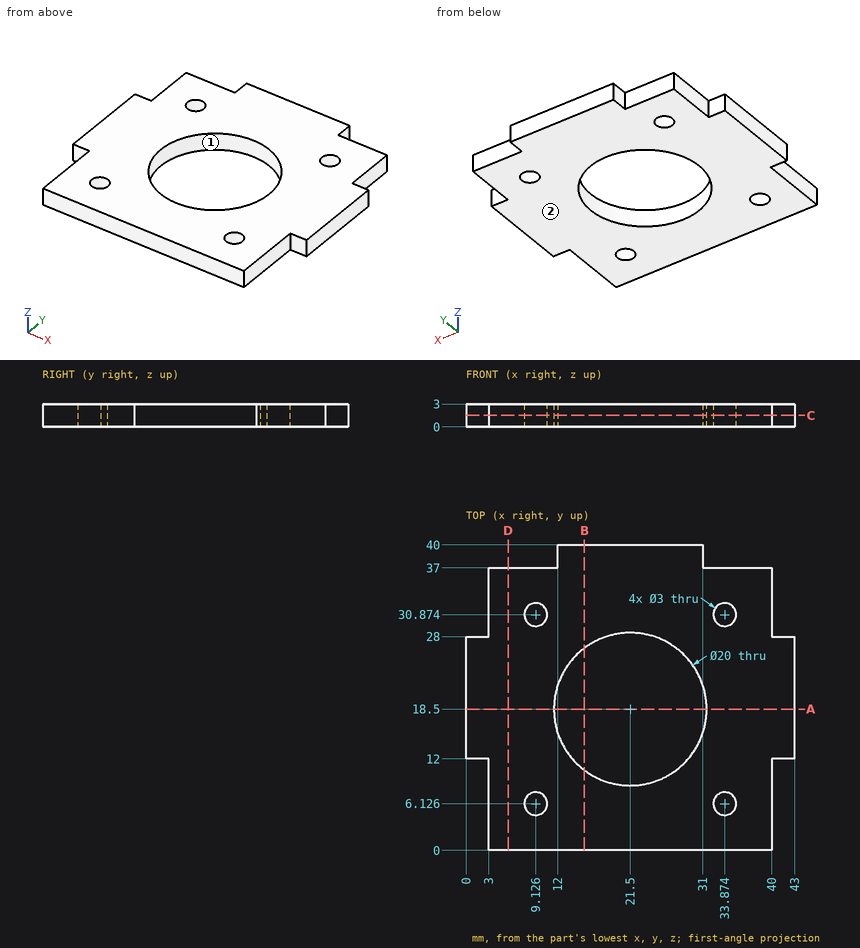
Input: dimensioned drawing with shaded views. Units: mm. Origin: part minimum x, y, z. Round coordinates to 2 decimals unless told otherwise and drop trailing zeros. Loops run counter-clockwise (first coordinate to the right, second up) from the corner with the lowest first, then second, coordinate; pieces in that order, holes last.
1) Pull-direction query (X, two-part tool) for the marked faces 1 and 2; classes: released by +X, released by -X, zero draft, split by the parting line, or undercut.
Ans:
face 1: undercut
face 2: zero draft
2) Pin query (flat end, axial travel): pin 1 (1.5 mm diameter, centred on x = 1.5, z = 1.5, fed in from -Y); pin 2 (1.5 mm diameter, centred on y = 38, z = 1.5, fed in from +X); pin 3 (0.9 mm diameter, centred on y = 5.5, z = 2, fed in from +X). Return the tip coordinate at first contact, or that it passes through.
Ans:
pin 1: stops at y = 12
pin 2: stops at x = 31
pin 3: stops at x = 40
3) Section query A-A on y = 18.5. Return the cut outline in (x, z), plus the area to 3 significant figures.
Ans:
outline: (0, 0) - (11.5, 0) - (11.5, 3) - (0, 3) - close; (31.5, 0) - (43, 0) - (43, 3) - (31.5, 3) - close
area: 69.0 mm2
4) Section query C-C on z = 1.5. Return the cut outline in (x, y) (1 decimal).
Ans:
outline: (0, 12) - (3, 12) - (3, 0) - (40, 0) - (40, 12) - (43, 12) - (43, 28) - (40, 28) - (40, 37) - (31, 37) - (31, 40) - (12, 40) - (12, 37) - (3, 37) - (3, 28) - (0, 28) - close; hole circle Ø3 at (9.1, 6.1); hole circle Ø3 at (9.1, 30.9); hole circle Ø20 at (21.5, 18.5); hole circle Ø3 at (33.9, 6.1); hole circle Ø3 at (33.9, 30.9)
5) Section query D-D on x = 5.5. Return the cut outline in (y, z).
Ans:
outline: (0, 0) - (37, 0) - (37, 3) - (0, 3) - close
6) Material intervals for line 1 (Y direction, x = 34, z = 2.05); line 2 (X direction, y = 5, z = 1.7) (1 decimal); line 3 (X direction, y = 30, z = 0.3) (1 decimal), sorted ascending.
Ans:
line 1: y = 0 to 4.63, 7.62 to 29.38, 32.37 to 37
line 2: x = 3 to 8.1, 10.1 to 32.9, 34.9 to 40
line 3: x = 3 to 7.9, 10.3 to 32.7, 35.1 to 40
7) Section query B-B on x = 15.5. Return the cut outline in (y, z), plus the area to 3 significant figures.
Ans:
outline: (0, 0) - (10.5, 0) - (10.5, 3) - (0, 3) - close; (26.5, 0) - (40, 0) - (40, 3) - (26.5, 3) - close
area: 72.0 mm2
